from build123d import *

# Parameters (mm, degrees)
BOSS_EXTRUDE1_DEPTH = 5
BOSS_EXTRUDE2_DEPTH = 35
BOSS_EXTRUDE3_DEPTH = 5


with BuildPart() as part:
    # Sketch1 → Boss-Extrude1 (new body)
    with BuildSketch(Plane(origin=(0, 0, 0), x_dir=(1, 0, 0), z_dir=(0, 1, 0))):
        with BuildLine():
            Line((-121.5, 46.952098291), (-70.985786928, -75))
            Line((-70.985786928, -75), (70.985786928, -75))
            Line((70.985786928, -75), (121.5, 46.952098291))
            ThreePointArc((121.5, 46.952098291), (0, 68.717806969), (-121.5, 46.952098291))
        make_face()
    extrude(amount=BOSS_EXTRUDE1_DEPTH)

    # Sketch2 → Boss-Extrude2 (add)
    with BuildSketch(Plane(origin=(0, 5, 0), x_dir=(1, 0, 0), z_dir=(0, 1, 0))):
        with BuildLine():
            Line((-48.833229971, 2.175293041), (-40.133863978, -18.826834324))
            ThreePointArc((-40.133863978, -18.826834324), (-36.450770983, -23.314696123), (-30.895068653, -25))
            Line((-30.895068653, -25), (30.895068653, -25))
            ThreePointArc((30.895068653, -25), (36.450770983, -23.314696123), (40.133863978, -18.826834324))
            Line((40.133863978, -18.826834324), (48.833229971, 2.175293041))
            ThreePointArc((48.833229971, 2.175293041), (48.269800459, 10.975861174), (40.959759978, 15.90848324))
            ThreePointArc((40.959759978, 15.90848324), (0, 18.717806969), (-40.959759978, 15.90848324))
            ThreePointArc((-40.959759978, 15.90848324), (-48.269800459, 10.975861174), (-48.833229971, 2.175293041))
        make_face()
    extrude(amount=BOSS_EXTRUDE2_DEPTH)

    # Sketch3 → Boss-Extrude3 (add)
    with BuildSketch(Plane(origin=(0, 40, 0), x_dir=(1, 0, 0), z_dir=(0, 1, 0))):
        with BuildLine():
            Line((-121.5, 46.952098291), (-70.985786928, -75))
            Line((-70.985786928, -75), (70.985786928, -75))
            Line((70.985786928, -75), (121.5, 46.952098291))
            ThreePointArc((121.5, 46.952098291), (0, 68.717806969), (-121.5, 46.952098291))
        make_face()
    extrude(amount=BOSS_EXTRUDE3_DEPTH)


solid = part.part
Check sheet for the modelled part. Datum: model origin and axes. Units: mm. A direction names the side the tool comes from. Give positions to 0.01 mm unless a question says otherwise; leave off trailing zeros. Loops run counter-clockwise (first coordinate to the right, second up) from the corner with the lowest first, then second, coordinate; pieces in that order, holes last. Notation, with made-up numbers: M 81.5,27.5 L 124.5,27.5 A15 ccw 124.5,52.5 Z; hole C 78.5,6.25 d10. An arc over 180 degrees is marked long. Use a Markdown table: item, result. Add a question column.
Q1. Sectioned sample at B-B, the plane y = 17.5. Record the cut outline in (x, z).
Q2. Go/stop test with flat-tipped pins: pin 1 (10 mm diameter, centred on x = 7, y = 34.5, fed in from +Z); pin 2 (6 mm diameter, centred on y = 24.5, z = -16.5, fed in from +X). Record where each tip stops, or that it passes through.
Q3. Sectioned sample at A-A, the plane z = -39.5. Record the cut outline in (x, y).
Q4. Scan lines: line 1 along Y through (x, z) = (79, 28); line 2 along Z through (x, y) = (19, 26); line 3 along Z through (x, y) = (-27, 7). Record each from-to range of solid material in increasing order. Write a range as [from, to].
Q5. Mould release check, pull along Y, two halves, no side actions. Record for faces 1 (the cylindrical face through (-36.52, 22.26, 23.27)), 2 (the flat face through (-96.596, 42.465, 13.17)), 3 (the flat face through (-2, 45, 2)): pulls with the +Y half, pulls with the -Y half, needs draft (parallel to the pull), parting line crosses it, or undercut.
Q6. Sectioned sample at D-D, the plane z = 0.5. Record the cut outline in (x, y).
Q7. Sectioned sample at C-C, the plane x = 105. Record the cut outline in (y, z).
Q8. Tool access check on faces 4 (the flat face through (-44.544, 22.255, 8.179)), 5 (the cylindrical face through (48.333, 22.255, -10.865)), 6 (the flat face through (44.423, 22.255, 8.473)), 7 (the flat face through (0, 22, 25)). Record the directions out of +Z, -Z, +X, -X, +Y, -Y that give a thin tool (end or side, any length) a straight path to the whole face; none if there is none.
Verdict:
| question | item | result |
|---|---|---|
| 1 | outline | M -48.83,-2.18 A10 ccw -40.96,-15.91 A300 ccw 40.96,-15.91 A10 ccw 48.83,-2.18 L 40.13,18.83 A10 ccw 30.9,25 L -30.9,25 A10 ccw -40.13,18.83 Z |
| 2 | pin 1 | z = 25 |
| 2 | pin 2 | x = 46.21 |
| 3 | outline | M -118.41,0 L 118.41,0 L 118.41,5 L -118.41,5 Z; M -118.41,40 L 118.41,40 L 118.41,45 L -118.41,45 Z |
| 4 | line 1 | [0, 5], [40, 45] |
| 4 | line 2 | [-18.12, 25] |
| 4 | line 3 | [-17.5, 25] |
| 5 | face 1 | undercut |
| 5 | face 2 | needs draft |
| 5 | face 3 | pulls with the +Y half |
| 6 | outline | M -101.84,0 L 101.84,0 L 101.84,5 L 47.73,5 L 47.73,40 L 101.84,40 L 101.84,45 L -101.84,45 L -101.84,40 L -47.73,40 L -47.73,5 L -101.84,5 Z |
| 7 | outline | M 0,-52.6 L 5,-52.6 L 5,-7.12 L 0,-7.12 Z; M 40,-52.6 L 45,-52.6 L 45,-7.12 L 40,-7.12 Z |
| 8 | face 4 | +Z, -X |
| 8 | face 5 | +X |
| 8 | face 6 | +Z, +X |
| 8 | face 7 | +Z, +X, -X |
